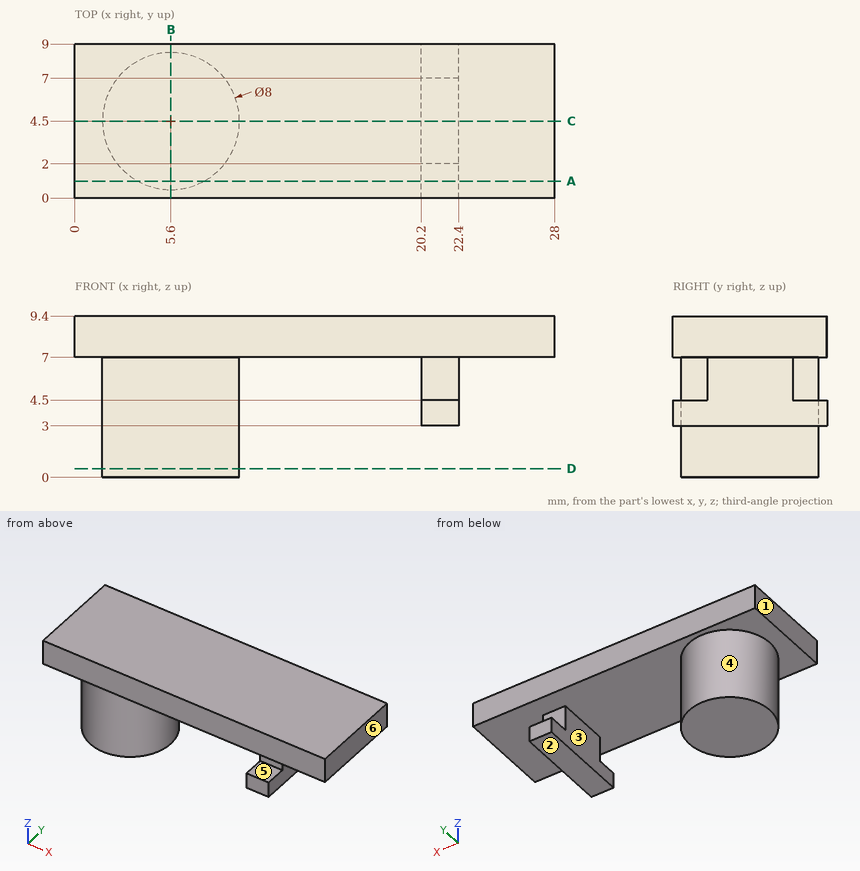
Job drawing, mm, ordinate dimensions from the low corner. One solid piece. A direction names the side the tool comes from. Round coordinates to 2 decimals unless told otherwise and drop trailing zeros. Order: outer loops, then holes, each group sorted by start corner. A loop starts at its lowest first (then second) coordinate and runs counter-clockwise, first axis right, second up. Notation, with made-up numbers: M 84,-9.5 L 123,-9.5 A37 ccw 123,29.5 Z; hole C -17.5,13.5 d9. An arc over 180 degrees is marked long. Write each question's results on one line, items separated by ' | '. Start each with the question number.
(1) Saw through at B-B, the plane x = 5.6. Give the cut face in (y, z).
(2) Saw through at A-A, the plane y = 1. Give the cut face in (x, z), then the cut area to 3 significant figures.
(3) Which spindle directions (+Z, -Z, +X, -X, +Y, -Y) get a long thin tool onto all of the face, cutting with end or side? Do the marked faces 4, 5 and 6. Say none if no direction does.
(4) Two-plate mould, pull along X, no slides. Class the marked faces 1, 2 and 3: pulls with the +X half, pulls with the -X half, needs draft (parallel to the pull), parting line crosses it, or undercut.
(5) Drop flat-ended pins along their axis: pin 1 (1.5 mm diameter, centred on y = 1.5, z = 6, fed in from -X); pin 2 (1.8 mm diameter, centred on x = 21, y = 5, fed in from -Z); pin 3 (0.7 mm diameter, centred on x = 21.5, z = 5.5, fed in from +Y); pin 4 (2.5 mm diameter, centred on x = 21, z = 5.5, fed in from -Y). Give the stop position or say it passes through.
(6) Saw through at D-D, the plane z = 0.5. Give the cut face in (x, y), then the cut area to 3 significant figures.
(7) Saw through at C-C, the plane y = 4.5. Give the cut face in (x, z).
(8) Probe probe 1 along Z at (x, y) = (15, 3.5); probe 2 along X at (y, z) = (3, 5); probe 3 along X at (y, z) = (5.5, 6.25). List the from-to ranges inside material, lowest first. Write a range as from..to.
Established:
1) outline: M 0,7 L 0.5,7 L 0.5,0 L 8.5,0 L 8.5,7 L 9,7 L 9,9.4 L 0,9.4 Z
2) outline: M 0,7 L 3.66,7 L 3.66,0 L 7.54,0 L 7.54,7 L 28,7 L 28,9.4 L 0,9.4 Z; M 20.2,3 L 22.4,3 L 22.4,4.5 L 20.2,4.5 Z | area: 97.6 mm^2
3) face 4: -Z | face 5: +X, -Y | face 6: +Z, -Z, +X, +Y, -Y
4) face 1: pulls with the -X half | face 2: needs draft | face 3: undercut
5) pin 1: stops at x = 2.29 | pin 2: stops at z = 3 | pin 3: stops at y = 7 | pin 4: stops at y = 0
6) outline: C 5.6,4.5 d8 | area: 50.3 mm^2
7) outline: M 0,7 L 1.6,7 L 1.6,0 L 9.6,0 L 9.6,7 L 20.2,7 L 20.2,3 L 22.4,3 L 22.4,7 L 28,7 L 28,9.4 L 0,9.4 Z
8) probe 1: z = 7..9.4 | probe 2: x = 1.89..9.31, 20.2..22.4 | probe 3: x = 1.73..9.47, 20.2..22.4
